Geometry: final body of the model. Coordinates: model frame, mm. Round coordinates to 2 decimals unless told otherwise and drop trailing zeros. Loops run counter-clockwise (first coordinate to the right, second up) from the corner with the lowest first, then second, coordinate; pieces in that order, holes last. Notation, with made-up numbers: (-16.75, 64) - (28.25, 64) arc R17 ccw to (28.25, 81) - close; hole circle Ø2 at (6.25, 37.5). An arc over 180 degrees is marked (long way). Write item = value, one per line. Start each with the question number.
Item 1: Section B-B (z = 0.75). Return loops of the section in (x, y), plus the area to 3 significant figures.
Item 2: Section A-A (y = 0). Return loops of the section in (x, z).
Item 3: Line query: line 1 (X direction, y = -0.15, z = 2.7); line 2 (Y direction, x = -2.05, z = 2.35); line 3 (X direction, y = 0.5, z = 3.6). Output: solid intervals per line, ascending. Write a range as from..to.
Item 4: Draft query along X for faces 1 (the cylindrical face through (-27.5, -0.1, 2.4)), 2 (the flat face through (0, 0, 4.8)), 3 (the cylindrical face through (23.82, -1.08, 2.37)), 4 (the cylindrical face through (-3.53, 0.61, 2.43)). Return one class per face: pulls with the +X half, pulls with the -X half, needs draft (parallel to the pull), parting line crosses it, or undercut.
Item 5: Section C-C (x = -2.05). Return loops of the section in (y, z), plus the area to 3 significant figures.
Autodesk Fusion 360 part; units mm, degrees
sketch "스케치1" plane through (0, 0, 0) normal (0, 0, 1) x (1, 0, 0)
  line L0 (-25, -2.5) -> (25, -2.5)
  arc A0 (25, -2.5) -> (25, 2.5) centre (25, 0) ccw
  line L1 (25, 2.5) -> (-25, 2.5)
  arc A1 (-25, 2.5) -> (-25, -2.5) centre (-25, 0) ccw
  line L2 (-25, 0) -> (25, 0) construction
  circle A2 centre (25, 0) radius 1.6
  circle A3 centre (-25, 0) radius 1.6
  dimension "d1" = 5
  dimension "d2" = 3.2
  dimension "d3" = 3.2
extrude "돌출1" add sketch "스케치1" along normal blind 4.8
sketch "스케치2" plane through (0, 0, 4.8) normal (0, 0, 1) x (-1, 0, 0)
  circle A0 centre (-25, 0) radius 1.6
  circle A1 centre (25, 0) radius 1.6
  arc A2 (25, -2.5) -> (25, 2.5) centre (25, 0) ccw
  line L0 (25, 2.5) -> (-25, 2.5)
  arc A3 (-25, 2.5) -> (-25, -2.5) centre (-25, 0) ccw
  line L1 (-25, -2.5) -> (25, -2.5)
  line L2 (2.05, -15) -> (2.05, 10)
  circle A4 centre (2.05, 0) radius 1.6
  dimension "d7" = 3.2
  dimension "d10" = 27.05
extrude "돌출2" cut sketch "스케치2" against normal blind 5 contours L2 A4 | L2 A4
Taken from the geometry:
q1.outline = (-25, -2.5) - (25, -2.5) arc R2.5 ccw to (25, 2.5) - (-25, 2.5) arc R2.5 ccw to start; hole circle Ø3.2 at (-25, 0); hole circle Ø3.2 at (-2.05, 0); hole circle Ø3.2 at (25, 0)
q1.area = 246 mm^2
q2.outline = (-27.5, 0) - (-26.6, 0) - (-26.6, 4.8) - (-27.5, 4.8) - close; (-23.4, 0) - (-3.65, 0) - (-3.65, 4.8) - (-23.4, 4.8) - close; (-0.45, 0) - (23.4, 0) - (23.4, 4.8) - (-0.45, 4.8) - close; (26.6, 0) - (27.5, 0) - (27.5, 4.8) - (26.6, 4.8) - close
q3.line_1 = -27.5..-26.59, -23.41..-3.64, -0.46..23.41, 26.59..27.5
q3.line_2 = -2.5..-1.6, 1.6..2.5
q3.line_3 = -27.45..-26.52, -23.48..-3.57, -0.53..23.48, 26.52..27.45
q4.face_1 = pulls with the -X half
q4.face_2 = needs draft
q4.face_3 = undercut
q4.face_4 = undercut
q5.outline = (-2.5, 0) - (-1.6, 0) - (-1.6, 4.8) - (-2.5, 4.8) - close; (1.6, 0) - (2.5, 0) - (2.5, 4.8) - (1.6, 4.8) - close
q5.area = 8.64 mm^2
